from build123d import *

# Parameters (mm, degrees)
SKETCH1_W           = 38.1
SKETCH1_H           = 25.4
BOSS_EXTRUDE1_DEPTH = 12.7
SKETCH2_R           = 6.35
CUT_EXTRUDE1_DEPTH  = 27.181720723
SKETCH3_R           = 3.175
CUT_EXTRUDE2_DEPTH  = 35.195796525


with BuildPart() as part:
    # Sketch1 → Boss-Extrude1 (new body)
    with BuildSketch(Plane(origin=(0, 0, 0), x_dir=(1, 0, 0), z_dir=(0, 1, 0))):
        Rectangle(SKETCH1_W, SKETCH1_H)
    extrude(amount=BOSS_EXTRUDE1_DEPTH)

    # Sketch2 → Cut-Extrude1 (cut, through all)
    with BuildSketch(Plane(origin=(0, 12.7, 0), x_dir=(1, 0, 0), z_dir=(0, 1, 0))):
        with Locations(Location((0, 0, 0), (0, 0, 270))):
            Circle(SKETCH2_R)
    extrude(amount=-CUT_EXTRUDE1_DEPTH, mode=Mode.SUBTRACT)

    # Sketch3 → Cut-Extrude2 (cut, through all)
    with BuildSketch(Plane(origin=(0, 0, -12.7), x_dir=(-1, 0, 0), z_dir=(0, 0, -1))):
        with Locations((-12.7, 6.35)):
            Circle(SKETCH3_R)
        with Locations(Location((12.7, 6.35, 0), (0, 0, 180))):
            Circle(SKETCH3_R)
    extrude(amount=-CUT_EXTRUDE2_DEPTH, mode=Mode.SUBTRACT)


solid = part.part
Source: CAD feature listing. Evaluate the final solid. Frame: model axes, mm. Give positions to 0.01 mm unless a question says otherwise; leave off trailing zeros. Write each loop counter-clockwise with the first axis right and the second up, starting at its lowest first coordinate (ties: lowest second). Pieces come first, ordered by that corner, then holes. Notation, with made-up numbers: (16, 76.25) -> (27, 76.25) arc R21 cw to (27, 91.25) -> close; hole circle Ø4 at (36.25, -14.75). An arc over 180 degrees is marked (long way). Write item = value, one per line.
Q1. Cut plane B-B on z = 0. Return loops of the section in (x, y) (3 decimals), then the cut area to 3 significant figures.
Here are the results:
outline = (-19.05, 0) -> (-6.35, 0) -> (-6.35, 12.7) -> (-19.05, 12.7) -> close; (6.35, 0) -> (19.05, 0) -> (19.05, 12.7) -> (6.35, 12.7) -> close; hole circle Ø6.35 at (-12.7, 6.35); hole circle Ø6.35 at (12.7, 6.35)
area = 259 mm²
Q2. Cut plane D-D on y = 2.5. Return loops of the section in (x, z).
Here are the results:
outline = (-19.05, -12.7) -> (19.05, -12.7) -> (19.05, 12.7) -> (-19.05, 12.7) -> close; hole circle Ø12.7 at (0, 0)
Q3. First-contact query: pin 1 (4 mm diameter, centred on x = -12.7, y = 6.35, fed in from -Z). Flat tip, straight axial feed; report the tip coordinate or a pass-through.
Here are the results:
pin_1 = through
Q4. Mould query, pull axis X, two halves, no side actions, for faces 1 (the face through (19.05, 6, 0)), 2 (the face through (4, 0, -6)), 3 (the face through (-3.86, 6.44, -5.04)). Classes: +X half, -X half, draft (parallel to the pull), parting line (faces both ways), or undercut.
Here are the results:
face_1 = +X half
face_2 = draft
face_3 = undercut
Q5. Cut plane C-C on x = 0. Return loops of the section in (y, z).
Here are the results:
outline = (0, -12.7) -> (12.7, -12.7) -> (12.7, -6.35) -> (0, -6.35) -> close; (0, 6.35) -> (12.7, 6.35) -> (12.7, 12.7) -> (0, 12.7) -> close
Q6. Cut plane A-A on y = 6.35. Return loops of the section in (x, z) (3 decimals).
Here are the results:
outline = (-19.05, -12.7) -> (-15.875, -12.7) -> (-15.875, 12.7) -> (-19.05, 12.7) -> close; (-9.525, -12.7) -> (9.525, -12.7) -> (9.525, 12.7) -> (-9.525, 12.7) -> close; (15.875, -12.7) -> (19.05, -12.7) -> (19.05, 12.7) -> (15.875, 12.7) -> close; hole circle Ø12.7 at (0, 0)
Q7. Line query: line 1 (Y direction, x = 12.7, z = 5) (3 decimals); line 2 (X direction, y = 7.25, z = 0); line 3 (X direction, y = 5.75, z = 10.25). Output: solid intervals per line, ascending. Write a range as from..to.
Here are the results:
line_1 = 0..3.175, 9.525..12.7
line_2 = -19.05..-15.74, -9.66..-6.35, 6.35..9.66, 15.74..19.05
line_3 = -19.05..-15.82, -9.58..9.58, 15.82..19.05
